Answer from the drawing. Dimensions are ordinates in mm from the lowest x, y and z of the part. A direction names the side the tool comes from. Coordinates: 2 decimals unless noted, no trailing zeros. Write each loop counter-clockwise with the first axis right and the second up, starting at its lowest first coordinate (ties: lowest second). Pieces come first, ordered by that corner, then holes. Notation, with made-up numbers: (-25, 57.5) - (4, 57.5) arc R23 cw to (4, 91.5) - close; hole circle Ø1 at (46.5, -37). An arc over 180 degrees is marked (long way). Use a Markdown table: item, result.
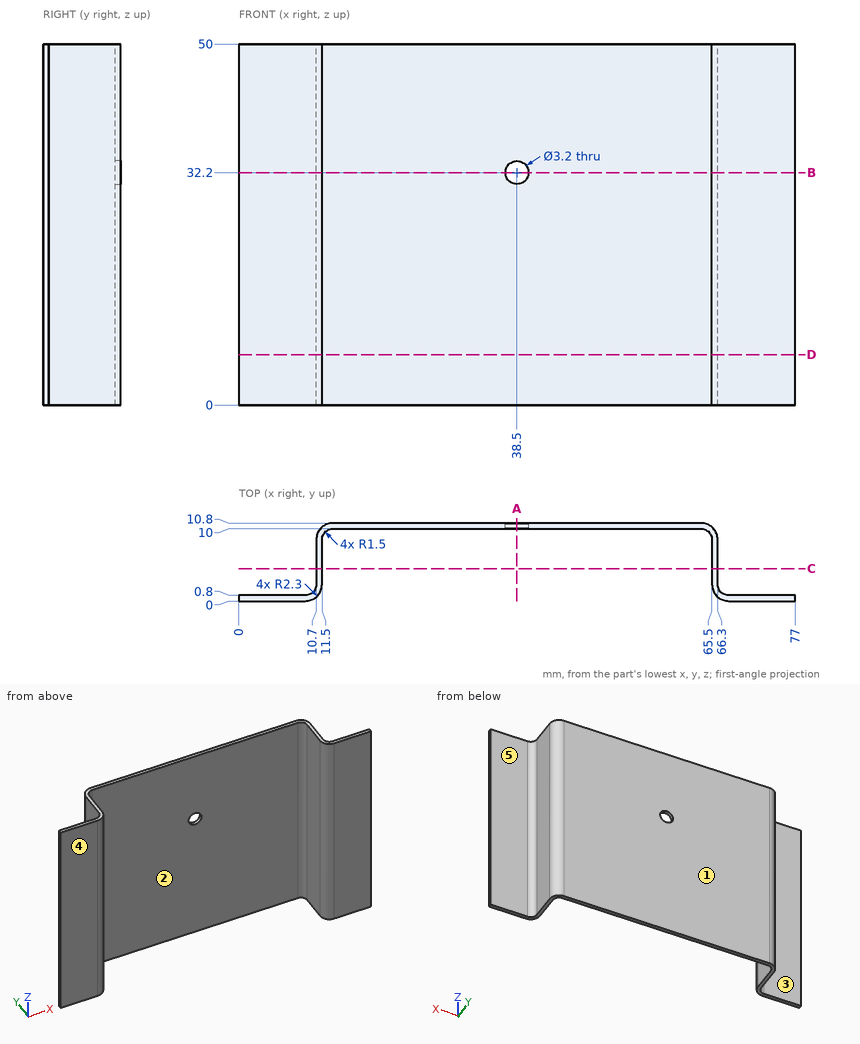
(1) A cutting plane is placed at A-A, the plane x = 38.5. Write down the section's boundary in (y, z), and give its area (3 significant figures).
Report:
| item | result |
|---|---|
| outline | (10, 0) - (10.8, 0) - (10.8, 30.6) - (10, 30.6) - close; (10, 33.8) - (10.8, 33.8) - (10.8, 50) - (10, 50) - close |
| area | 37.4 mm² |
(2) A cutting plane is placed at D-D, the plane z = 7. Write down the section's boundary in (x, y).
Report:
| item | result |
|---|---|
| outline | (0, 0) - (9.2, 0) arc R2.3 ccw to (11.5, 2.3) - (11.5, 8.5) arc R1.5 cw to (13, 10) - (64, 10) arc R1.5 cw to (65.5, 8.5) - (65.5, 2.3) arc R2.3 ccw to (67.8, 0) - (77, 0) - (77, 0.8) - (67.8, 0.8) arc R1.5 cw to (66.3, 2.3) - (66.3, 8.5) arc R2.3 ccw to (64, 10.8) - (13, 10.8) arc R2.3 ccw to (10.7, 8.5) - (10.7, 2.3) arc R1.5 cw to (9.2, 0.8) - (0, 0.8) - close |
(3) Straight lines are drawn through the part: L1, parallel to X at y = 2.25, z = 18.5; L2, parallel to Y at x = 41.5, z = 40; L3, parallel to Y at x = 6, z = 13.5. For each, find the intervals that lie inside material, in ascending order.
Report:
| item | result |
|---|---|
| L1 | x = 10.7 to 11.5, 65.5 to 66.3 |
| L2 | y = 10 to 10.8 |
| L3 | y = 0 to 0.8 |
(4) The mould has two halves that part along X. Classify the marked faces 1 and 2: pulls with the +X half, pulls with the -X half, needs draft (parallel to the pull), parting line crosses it, or undercut.
Report:
| item | result |
|---|---|
| face 1 | needs draft |
| face 2 | undercut |
(5) A cutting plane is placed at C-C, the plane y = 4.5. Write down the section's boundary in (x, z).
Report:
| item | result |
|---|---|
| outline | (10.7, 0) - (11.5, 0) - (11.5, 50) - (10.7, 50) - close; (65.5, 0) - (66.3, 0) - (66.3, 50) - (65.5, 50) - close |
(6) A cutting plane is placed at B-B, the plane z = 32.2. Write down the section's boundary in (x, y).
Report:
| item | result |
|---|---|
| outline | (0, 0) - (9.2, 0) arc R2.3 ccw to (11.5, 2.3) - (11.5, 8.5) arc R1.5 cw to (13, 10) - (36.9, 10) - (36.9, 10.8) - (13, 10.8) arc R2.3 ccw to (10.7, 8.5) - (10.7, 2.3) arc R1.5 cw to (9.2, 0.8) - (0, 0.8) - close; (40.1, 10) - (64, 10) arc R1.5 cw to (65.5, 8.5) - (65.5, 2.3) arc R2.3 ccw to (67.8, 0) - (77, 0) - (77, 0.8) - (67.8, 0.8) arc R1.5 cw to (66.3, 2.3) - (66.3, 8.5) arc R2.3 ccw to (64, 10.8) - (40.1, 10.8) - close |
(7) Each of these flat-tipped pins is pushed along its axis until it touches: P1, Ø1, axis at x = 17.5, z = 38, coming from the -Y side; P2, Ø3, axis at y = 6, z = 24.5, coming from the +X side; P3, Ø5, axis at y = 7.5, z = 33, coming from the -X side; P4, Ø1.9, axis at x = 38.5, z = 32.2, coming from the +Y side. Where does it stop, or does it pass through?
Report:
| item | result |
|---|---|
| P1 | stops at y = 10 |
| P2 | stops at x = 66.3 |
| P3 | stops at x = 10.7 |
| P4 | passes through |
(8) For the marked faces 3, 4 and 5, determine the directions among +Z, -Z, +X, -X, +Y, -Y from which every point of the face is accessible in a straight line to the end or side of a thin tool.
Report:
| item | result |
|---|---|
| face 3 | +Z, -Z, -X, +Y |
| face 4 | +Z, -Z, +X, -X, -Y |
| face 5 | +Z, -Z, +X, +Y |
